Could you check a few things on this model? Use its own coordinates, in mm. A direction names the side the tool comes from. Round coordinates to 2 decimals unless told otherwise and drop trailing zeros. Loops run counter-clockwise (first coordinate to the right, second up) from the corner with the lowest first, then second, coordinate; pieces in that order, holes last. Notation, with made-up numbers: (43.5, -29) -> (82.5, -29) arc R27 cw to (82.5, -5) -> close; hole circle Ø5 at (-7, -14). An arc over 180 degrees is marked (long way). Write each question's results on one line, items separated by ' | '. Start each with the question number.
1) We'd pull the mould along X, two halves only. Please class faces 4 (the flat face through (-51.85, 18, 2)), 5 (the cylindrical face through (46.813, -36.543, 1.479)), 6 (the flat face through (2, 15, 9)): pulls with the +X half, pulls with the -X half, needs draft (parallel to the pull), parting line crosses it, or undercut.
2) Imagine slicing it at C-C, the plane y = -35.25. List the corners of the cut face in (x, z) for me (3 decimals), plus the area to 3 significant figures.
3) Imagine slicing it at B-B, the plane x = 14.55. List the corners of the cut face in (y, z) for me, plus the area to 4 significant figures.
4) Which directions (+Z, -Z, +X, -X, +Y, -Y) give clear straight access to the entire face, cutting with the end or side of a thin tool? Please do faces 1 (the flat face through (57, -20, 15)), 2 (the flat face through (5.1, -34, 8)), 3 (the cylindrical face through (-8.446, 39.038, 10.24)).
5) Imagine slicing it at D-D, the plane y = 1. List the corners of the cut face in (x, z) for me, plus the area to 3 significant figures.
6) For P1, Ø6, axis at y = -33.5, z = 9.5, coming from the +X side; P2, Ø1, axis at y = 17, z = 15.5, coming from the -X side; P3, Ø10, axis at y = -0.5, z = 9.5, coming from the -X side, each with a flat end and sliding along its axis, tell me the tip position at first contact or that it passes through.
7) If I drill on probe 1 along X at (y, z) = (-25, 15.75); probe 2 along Y at (x, z) = (46, 11.25); probe 3 along Y at (x, z) = (1, 9.5), over which ranges is the centre line in solid material (lowest first)?
8) Imagine slicing it at A-A, the plane y = 28. List the corners of the cut face in (x, z) for me.
from build123d import *

# Parameters (mm, degrees)
F0_R      = 1.325
F1_DEPTH  = 3
F2_R      = 2.625
F2_R_2    = 1.5
F3_DEPTH  = 8
F4_R      = 3.5
F5_DEPTH  = 6.5
F7_DEPTH  = 7.5
F8_W      = 4
F8_H      = 75
F9_DEPTH  = 10
F10_W     = 4
F10_H     = 75
F11_DEPTH = 10
F13_DEPTH = 10
F14_W     = 30
F14_H     = 17.5
F15_DEPTH = 64.001
F16_W     = 4
F16_H     = 2.5
F17_DEPTH = 79.751
F20_DEPTH = 3.001
F18_W     = 48.9
F18_H     = 5
F21_DEPTH = 7.5
F23_DEPTH = 3.001
F24_W     = 4
F24_H     = 2.5
F25_DEPTH = 79.751
F26_DEPTH = 9.501
F27_W     = 7
F27_H     = 30
F28_DEPTH = 7.5
F30_DEPTH = 2
F31_R     = 3.5
F32_DEPTH = 71.951
F33_R     = 3.5
F34_DEPTH = 123.101


# Not quite as in the source:
# - a fillet or chamfer that OpenCascade refuses, or shapes differently, is made with other operations: its cross-section is extruded or revolved along the edge and cut away or added


with BuildPart() as f1:
    # F0 (on Top) → F1 (new body)
    with BuildSketch(Plane.XY):
        with BuildLine():
            Line((57.1, 42.25), (0, 42.25))
            Line((0, 42.25), (-57.1, 42.25))
            ThreePointArc((-57.1, 42.25), (-60.6355339059, 40.7855339059), (-62.1, 37.25))
            Line((-62.1, 37.25), (-62.1, 0))
            Line((-62.1, 0), (-62.1, -37.25))
            ThreePointArc((-62.1, -37.25), (-60.6355339059, -40.7855339059), (-57.1, -42.25))
            Line((-57.1, -42.25), (0, -42.25))
            Line((0, -42.25), (57.1, -42.25))
            ThreePointArc((57.1, -42.25), (60.6355339059, -40.7855339059), (62.1, -37.25))
            Line((62.1, -37.25), (62.1, 0))
            Line((62.1, 0), (62.1, 37.25))
            ThreePointArc((62.1, 37.25), (60.6355339059, 40.7855339059), (57.1, 42.25))
        make_face()
        with Locations((-47.1, -35.25)):
            Circle(F0_R, mode=Mode.SUBTRACT)
        with Locations((47.1, -35.25)):
            Circle(F0_R, mode=Mode.SUBTRACT)
        with Locations((-47.1, 35.25)):
            Circle(F0_R, mode=Mode.SUBTRACT)
        with Locations((47.1, 35.25)):
            Circle(F0_R, mode=Mode.SUBTRACT)
    extrude(amount=F1_DEPTH)

    # F2 (on face) → F3 (join)
    with BuildSketch(Plane.XY.offset(3)):
        with Locations((-56.1, -27.85)):
            Circle(F2_R)
        with Locations((-56.1, -27.85)):
            Circle(F2_R_2, mode=Mode.SUBTRACT)
        with Locations((-7.71, -27.85)):
            Circle(F2_R)
        with Locations((-7.71, -27.85)):
            Circle(F2_R_2, mode=Mode.SUBTRACT)
        with Locations((-52.86, 38.25)):
            Circle(F2_R)
        with Locations((-52.86, 38.25)):
            Circle(F2_R_2, mode=Mode.SUBTRACT)
        with Locations((-10.95, 38.25)):
            Circle(F2_R)
        with Locations((-10.95, 38.25)):
            Circle(F2_R_2, mode=Mode.SUBTRACT)
    extrude(amount=F3_DEPTH)

    # F4 (on face) → F5 (join)
    with BuildSketch(Plane.XY.offset(3)):
        with Locations((-10.95, 38.25)):
            Circle(F4_R)
        with Locations((-7.71, -27.85)):
            Circle(F4_R)
        with Locations((-56.1, -27.85)):
            Circle(F4_R)
        with Locations((-52.86, 38.25)):
            Circle(F4_R)
    extrude(amount=F5_DEPTH)

    # F6 (on face) → F7 (join)
    with BuildSketch(Plane.XY.offset(3)):
        Polygon((5.1, 37.5), (2.1, 37.5), (-1.9, 37.5), (-1.9, -37.5), (2.1, -37.5), (5.1, -37.5), align=None)
        Polygon((61, 37.5), (57, 37.5), (54, 37.5), (54, -37.5), (57, -37.5), (61, -37.5), align=None)
    extrude(amount=F7_DEPTH)

    # F8 (on face) → F9 (join)
    with BuildSketch(Plane.XY.offset(10.5)):
        with Locations((0.1, 0)):
            Rectangle(F8_W, F8_H)
    extrude(amount=F9_DEPTH)

    # F10 (on face) → F11 (join)
    with BuildSketch(Plane.XY.offset(10.5)):
        with Locations((59, 0)):
            Rectangle(F10_W, F10_H)
    extrude(amount=F11_DEPTH)

    # F12 (on face) → F13 (cut)
    with BuildSketch(Plane.XY.offset(20.5)):
        Polygon((60, -25.1), (57, -25.1), (57, -29.3), (60, -29.3), (60, -27.2), align=None)
        Polygon((60, 27.2), (60, 29.3), (57, 29.3), (57, 25.1), (60, 25.1), align=None)
    extrude(amount=-F13_DEPTH, mode=Mode.SUBTRACT)

    # F14 (on face) → F15 (cut, through all)
    with BuildSketch(Plane(origin=(-1.9, 0, 0), x_dir=(0, -1, 0), z_dir=(-1, 0, 0))):
        with Locations((0, 11.75)):
            Rectangle(F14_W, F14_H)
    extrude(amount=-F15_DEPTH, mode=Mode.SUBTRACT)

    # F16 (on face) → F17 (cut, through all)
    with BuildSketch(Plane.XZ.offset(37.5)):
        with Locations((0.1, 19.25)):
            Rectangle(F16_W, F16_H)
    extrude(amount=-F17_DEPTH, mode=Mode.SUBTRACT)

    # F19 (on face) → F20 (cut, through all)
    with BuildSketch(Plane.XY.offset(3)):
        with BuildLine():
            Line((47.1, 20), (12.1, 20))
            ThreePointArc((12.1, 20), (8.5644660941, 18.5355339059), (7.1, 15))
            Line((7.1, 15), (7.1, -15))
            ThreePointArc((7.1, -15), (8.5644660941, -18.5355339059), (12.1, -20))
            Line((12.1, -20), (47.1, -20))
            ThreePointArc((47.1, -20), (50.6355339059, -18.5355339059), (52.1, -15))
            Line((52.1, -15), (52.1, 15))
            ThreePointArc((52.1, 15), (50.6355339059, 18.5355339059), (47.1, 20))
        make_face()
    extrude(amount=-F20_DEPTH, mode=Mode.SUBTRACT)

    # F18 (on face) → F21 (join)
    with BuildSketch(Plane.XY.offset(3)):
        with Locations((29.55, -27.2)):
            Rectangle(F18_W, F18_H)
        with Locations((29.55, 27.2)):
            Rectangle(F18_W, F18_H)
    extrude(amount=F21_DEPTH)

    # F22 (on face) → F23 (cut, through all)
    with BuildSketch(Plane.XY.offset(3)):
        with BuildLine():
            Line((-16.85, 30), (-46.85, 30))
            ThreePointArc((-46.85, 30), (-50.3855339059, 28.5355339059), (-51.85, 25))
            Line((-51.85, 25), (-51.85, 10))
            ThreePointArc((-51.85, 10), (-50.3855339059, 6.4644660941), (-46.85, 5))
            Line((-46.85, 5), (-16.85, 5))
            ThreePointArc((-16.85, 5), (-13.3144660941, 6.4644660941), (-11.85, 10))
            Line((-11.85, 10), (-11.85, 25))
            ThreePointArc((-11.85, 25), (-13.3144660941, 28.5355339059), (-16.85, 30))
        make_face()
        with BuildLine():
            Line((-46.85, -30), (-16.85, -30))
            ThreePointArc((-16.85, -30), (-13.3144660941, -28.5355339059), (-11.85, -25))
            Line((-11.85, -25), (-11.85, -10))
            ThreePointArc((-11.85, -10), (-13.3144660941, -6.4644660941), (-16.85, -5))
            Line((-16.85, -5), (-46.85, -5))
            ThreePointArc((-46.85, -5), (-50.3855339059, -6.4644660941), (-51.85, -10))
            Line((-51.85, -10), (-51.85, -25))
            ThreePointArc((-51.85, -25), (-50.3855339059, -28.5355339059), (-46.85, -30))
        make_face()
    extrude(amount=-F23_DEPTH, mode=Mode.SUBTRACT)

    # F24 (on face) → F25 (cut, through all)
    with BuildSketch(Plane.XZ.offset(37.5)):
        with Locations((59, 19.25)):
            Rectangle(F24_W, F24_H)
    extrude(amount=-F25_DEPTH, mode=Mode.SUBTRACT)

    # F26 (cut, through all): faces of the model
    f26_faces = [f1.faces().sort_by_distance(p)[0] for p in [
        (-52.86, 38.25, 9.5),
        (-10.95, 38.25, 9.5),
        (-7.71, -27.85, 9.5),
        (-56.1, -27.85, 9.5),
    ]]
    extrude(f26_faces, amount=-F26_DEPTH, mode=Mode.SUBTRACT)

    # F27 (on face) → F28 (join)
    with BuildSketch(Plane.XY.offset(3)):
        with Locations((57.5, 0)):
            Rectangle(F27_W, F27_H)
    extrude(amount=F28_DEPTH)

    # F29: fillet of radius 1 on 4 edges, made by hand

    # F29_s1 → F29_t2 (revolve, cut)
    with BuildSketch(Plane.XZ.offset(-38.25)):
        with BuildLine():
            ThreePointArc((-49.36, 8.5078432584), (-49.61, 9.1692810861), (-50.235, 9.5))
            Line((-50.235, 9.5), (-49.36, 9.5))
            Line((-49.36, 9.5), (-49.36, 8.5078432584))
        make_face()
    revolve(axis=Axis((-52.86, 38.25, 9.5), (0, 0, 1)), mode=Mode.SUBTRACT)

    # F29_s3 → F29_t4 (revolve, cut)
    with BuildSketch(Plane.XZ.offset(-38.25)):
        with BuildLine():
            ThreePointArc((-7.45, 8.5078432584), (-7.7, 9.1692810861), (-8.325, 9.5))
            Line((-8.325, 9.5), (-7.45, 9.5))
            Line((-7.45, 9.5), (-7.45, 8.5078432584))
        make_face()
    revolve(axis=Axis((-10.95, 38.25, 9.5), (0, 0, 1)), mode=Mode.SUBTRACT)

    # F29_s5 → F29_t6 (revolve, cut)
    with BuildSketch(Plane.XZ.offset(27.85)):
        with BuildLine():
            ThreePointArc((-4.21, 8.5078432584), (-4.46, 9.1692810861), (-5.085, 9.5))
            Line((-5.085, 9.5), (-4.21, 9.5))
            Line((-4.21, 9.5), (-4.21, 8.5078432584))
        make_face()
    revolve(axis=Axis((-7.71, -27.85, 9.5), (0, 0, 1)), mode=Mode.SUBTRACT)

    # F29_s7 → F29_t8 (revolve, cut)
    with BuildSketch(Plane.XZ.offset(27.85)):
        with BuildLine():
            ThreePointArc((-52.6, 8.5078432584), (-52.85, 9.1692810861), (-53.475, 9.5))
            Line((-53.475, 9.5), (-52.6, 9.5))
            Line((-52.6, 9.5), (-52.6, 8.5078432584))
        make_face()
    revolve(axis=Axis((-56.1, -27.85, 9.5), (0, 0, 1)), mode=Mode.SUBTRACT)

    # F30 (add): a face of the model
    f30_faces = [f1.faces().sort_by_distance(p)[0] for p in [
        (3.6, -36.5463643253, 10.5),
    ]]
    extrude(f30_faces, amount=F30_DEPTH)

    # F31 (on face) → F32 (cut, through all)
    with BuildSketch(Plane.XZ.offset(29.7)):
        with Locations((29.55, 7.75)):
            Circle(F31_R)
        with Locations((14.55, 7.75)):
            Circle(F31_R)
        with Locations((44.55, 7.75)):
            Circle(F31_R)
    extrude(amount=-F32_DEPTH, mode=Mode.SUBTRACT)

    # F33 (on face) → F34 (cut, through all)
    with BuildSketch(Plane.YZ.offset(61)):
        with Locations((-8, 7.75)):
            Circle(F33_R)
        with Locations((8, 7.75)):
            Circle(F33_R)
    extrude(amount=-F34_DEPTH, mode=Mode.SUBTRACT)


solid = f1.part
Checked values:
1) face 4: undercut | face 5: undercut | face 6: needs draft
2) outline: (-62.1, 0) -> (-48.425, 0) -> (-48.425, 3) -> (-62.1, 3) -> close; (-45.775, 0) -> (45.775, 0) -> (45.775, 3) -> (5.1, 3) -> (5.1, 12.5) -> (2.1, 12.5) -> (2.1, 18) -> (-1.9, 18) -> (-1.9, 3) -> (-45.775, 3) -> close; (48.425, 0) -> (62.1, 0) -> (62.1, 3) -> (61, 3) -> (61, 18) -> (57, 18) -> (57, 12.5) -> (54, 12.5) -> (54, 3) -> (48.425, 3) -> close | area: 534 mm^2
3) outline: (-42.25, 0) -> (-20, 0) -> (-20, 3) -> (-24.7, 3) -> (-24.7, 4.25) -> (-29.7, 4.25) -> (-29.7, 3) -> (-42.25, 3) -> close; (-29.7, 11.25) -> (-24.7, 11.25) -> (-24.7, 12.5) -> (-29.7, 12.5) -> close; (20, 0) -> (42.25, 0) -> (42.25, 3) -> (29.7, 3) -> (29.7, 4.25) -> (24.7, 4.25) -> (24.7, 3) -> (20, 3) -> close; (24.7, 11.25) -> (29.7, 11.25) -> (29.7, 12.5) -> (24.7, 12.5) -> close | area: 158.5 mm^2
4) face 1: +Z, +Y, -Y | face 2: +Z, -Y | face 3: +Z
5) outline: (-62.1, 0) -> (7.1, 0) -> (7.1, 3) -> (-62.1, 3) -> close; (52.1, 0) -> (62.1, 0) -> (62.1, 3) -> (61, 3) -> (61, 12.5) -> (54, 12.5) -> (54, 3) -> (52.1, 3) -> close | area: 304 mm^2
6) P1: x = 61 | P2: x = -1.9 | P3: x = 54
7) probe 1: -1.9 to 2.1, 57 to 61 | probe 2: -29.7 to -24.7, 24.7 to 29.7 | probe 3: -37.5 to -15, 15 to 37.5
8) outline: (-62.1, 0) -> (-50.85, 0) -> (-50.85, 3) -> (-62.1, 3) -> close; (-12.85, 0) -> (62.1, 0) -> (62.1, 3) -> (61, 3) -> (61, 18) -> (60, 18) -> (60, 12.5) -> (2.1, 12.5) -> (2.1, 18) -> (-1.9, 18) -> (-1.9, 3) -> (-12.85, 3) -> close; hole circle Ø7 at (14.55, 7.75); hole circle Ø7 at (29.55, 7.75); hole circle Ø7 at (44.55, 7.75)
